The model under review builds one solid part; all positions refer to its coordinate system, in mm. Face numbers are marked on the shaded views. A direction names the side the tool comes from. Round coordinates to 2 decimals unless told otherwise and drop trailing zeros. Write each loop counter-clockwise with the first axis right and the second up, starting at its lowest first coordinate (ties: lowest second). Pieces come first, ordered by that corner, then holes. Notation, with made-up numbers: (-38, 8.5) - (8, 8.5) arc R25 cw to (8, 24.5) - close; hole circle Ø11 at (-5, 78). An arc over 180 degrees is marked (long way). Return JSON: item names as keys, results as strings.
from build123d import *

# Parameters (mm, degrees)
SKETCH1_R            = 4
BOSS_EXTRUDE1_DEPTH  = 100
SKETCH2_R            = 3
CUT_EXTRUDE1_DEPTH   = 101.159872204
SKETCH3_R            = 12.5
BOSS_EXTRUDE2_DEPTH  = 5
SKETCH9_W            = 5.5
SKETCH9_H            = 3
CUT_EXTRUDE2_DEPTH   = 22.5
SKETCH2_2_R          = 3
CUT_EXTRUDE3_DEPTH   = 103.743612972
BOSS_EXTRUDE6_DEPTH  = 1
SKETCH18_W           = 10
SKETCH18_H           = 17.5
BOSS_EXTRUDE10_DEPTH = 10
SKETCH19_R           = 3
BOSS_EXTRUDE11_DEPTH = 2.5


with BuildPart() as part:
    # Sketch1 → Boss-Extrude1 (new body)
    with BuildSketch(Plane(origin=(0, 0, 0), x_dir=(1, 0, 0), z_dir=(0, 1, 0))):
        with Locations(Location((0, 0, 0), (0, 0, 270))):
            Circle(SKETCH1_R)
    extrude(amount=BOSS_EXTRUDE1_DEPTH)

    # Sketch2 → Cut-Extrude1 (cut, through all)
    with BuildSketch(Plane(origin=(0, 100, 0), x_dir=(1, 0, 0), z_dir=(0, 1, 0))):
        with Locations(Location((0, 0, 0), (0, 0, 270))):
            Circle(SKETCH2_R)
    extrude(amount=-CUT_EXTRUDE1_DEPTH, mode=Mode.SUBTRACT)

    # Sketch3 → Boss-Extrude2 (add)
    with BuildSketch(Plane(origin=(0, 100, 0), x_dir=(1, 0, 0), z_dir=(0, 1, 0))):
        with Locations(Location((0, 0, 0), (0, 0, 270))):
            Circle(SKETCH3_R)
    extrude(amount=-BOSS_EXTRUDE2_DEPTH)

    # Sketch5 → Loft2 section 0
    with BuildSketch(Plane.XY):
        with BuildLine():
            Line((-12.5, 100), (12.5, 100))
            Line((12.5, 100), (12.5, 95))
            Line((12.5, 95), (-12.5, 95))
            Line((-12.5, 95), (-12.5, 100))
        make_face()
    # Sketch4 → Loft2 section 1
    with BuildSketch(Plane.XY.offset(20)):
        with BuildLine():
            Line((-3.75, 100), (3.75, 100))
            Line((3.75, 100), (3.75, 95))
            Line((3.75, 95), (-3.75, 95))
            Line((-3.75, 95), (-3.75, 100))
        make_face()
    loft()

    # Sketch9 → Cut-Extrude2 (cut)
    with BuildSketch(Plane.XY.offset(20)):
        with Locations((0, 97.5)):
            Rectangle(SKETCH9_W, SKETCH9_H)
    extrude(amount=-CUT_EXTRUDE2_DEPTH, mode=Mode.SUBTRACT)

    # Sketch2_2 → Cut-Extrude3 (cut, through all)
    with BuildSketch(Plane(origin=(0, 100, 0), x_dir=(1, 0, 0), z_dir=(0, 1, 0))):
        with Locations(Location((0, 0, 0), (0, 0, 270))):
            Circle(SKETCH2_2_R)
    extrude(amount=-CUT_EXTRUDE3_DEPTH, mode=Mode.SUBTRACT)

    # Sketch14 → Boss-Extrude6 (add)
    with BuildSketch(Plane(origin=(0, 100, 0), x_dir=(1, 0, 0), z_dir=(0, 1, 0))):
        Polygon((10.456538619, 0), (5.22826931, 9.05562808), (-5.22826931, 9.05562808), (-10.456538619, 0), (-5.22826931, -9.05562808), (5.22826931, -9.05562808), align=None)
    extrude(amount=BOSS_EXTRUDE6_DEPTH)

    # Sketch18 → Boss-Extrude10 (add)
    with BuildSketch(Plane.XY.offset(3)):
        with Locations((0, 46.25)):
            Rectangle(SKETCH18_W, SKETCH18_H)
    extrude(amount=BOSS_EXTRUDE10_DEPTH)

    # Sketch19 → Boss-Extrude11 (add)
    with BuildSketch(Plane.XY.offset(13)):
        with Locations(Location((0, 51.25, 0), (0, 0, 180))):
            Circle(SKETCH19_R)
        with Locations(Location((0, 41.25, 0), (0, 0, 180))):
            Circle(SKETCH19_R)
    extrude(amount=BOSS_EXTRUDE11_DEPTH)


solid = part.part
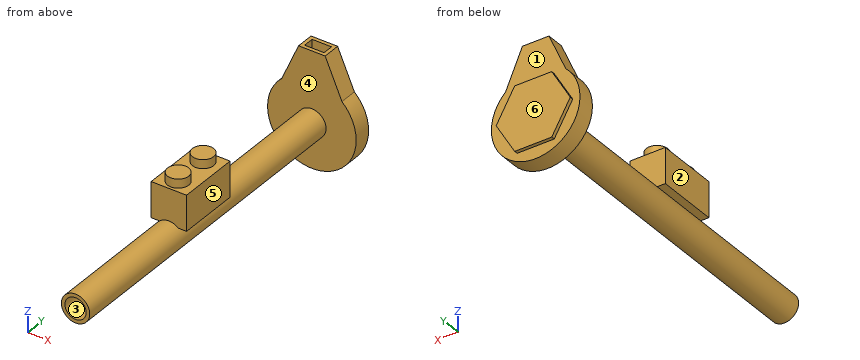
(1) Mouldability with a two-part tool opening along Y and no side actions: class the marked faces 4, 5 and 6 as released by +Y, released by -Y, zero draft, split by the parting line, or undercut.
Filled in:
{"face 4": "undercut", "face 5": "zero draft", "face 6": "released by +Y"}
(2) Add section D-D (x = 9.5). Write out the cut boundary in (y, z), plus the area to 3 significant figures.
Filled in:
{"outline": "(95, -8.12) - (100, -8.12) - (100, -1.66) - (101, -1.66) - (101, 1.66) - (100, 1.66) - (100, 8.12) - (95, 8.12) - close", "area": "84.6 mm2"}
(3) Add section A-A (y = 46). Write out the cut boundary in (x, z).
Filled in:
{"outline": "(-5, 3) - (-2.65, 3) arc R4 ccw (long way) to (2.65, 3) - (5, 3) - (5, 13) - (-5, 13) - close; hole circle Ø6 at (0, 0)"}
(4) For the marked faces 1, 2 and 3, list the 3-axis set-ups (+Z, -Z, +X, -X, +Y, -Y) from which the entire face can be reached by the end or side of a thin tool; tool diameter is ignored.
Filled in:
{"face 1": "+Y", "face 2": "+Z, -Z, -X, -Y", "face 3": "-Y"}
(5) Wall thickness on line 1 (X direction, y = 58.5, z = 0); line 2 (Y direction, x = -4.5, z = 3.5); line 3 (Y direction, x = 5, z = 0): over which ranges is each line inside the solid? List them lowest first.
Filled in:
{"line 1": "x = -4 to -3, 3 to 4", "line 2": "y = 37.5 to 55, 95 to 101", "line 3": "y = 95 to 101"}
(6) Add section C-C (z = 10.5). Write out the cut boundary in (x, y), plus the area to 3 significant figures.
Filled in:
{"outline": "(-7.91, 95) - (7.91, 95) - (7.91, 100) - (-7.91, 100) - close; (-5, 37.5) - (5, 37.5) - (5, 55) - (-5, 55) - close; hole (-2.75, 96) - (2.75, 96) - (2.75, 99) - (-2.75, 99) - close", "area": "238 mm2"}
(7) Clearance check with flat-ended pins moving along their axes: pin 1 Ø3.5 at (y, z) = (97, 10.5) entering from +X; pin 2 Ø3 at (x, y) = (-0.5, 42.5) entering from +Z; pin 3 Ø3 at (y, z) = (49, 6) entering from -X; pin 4 Ø1 at (x, y) = (-5.5, 69.5) entering from +Z. State where each tip first meets the part, or that it passes through.
Filled in:
{"pin 1": "stops at x = 8.93", "pin 2": "stops at z = 15.5", "pin 3": "stops at x = -5", "pin 4": "passes through"}
